Geometry check sheet. Reference: the model listing, model coordinates, mm. Coordinates: 2 decimals unless noted, no trailing zeros. Write each loop counter-clockwise with the first axis right and the second up, starting at its lowest first coordinate (ties: lowest second). Pieces come first, ordered by that corner, then holes.
Autodesk Inventor part; units mm, degrees
ref_plane "YZ Plane" through (0, 0, 0) normal (1, 0, 0) x (0, 1, 0)
ref_plane "XZ Plane" through (0, 0, 0) normal (0, 1, 0) x (-1, 0, 0)
ref_plane "XY Plane" through (0, 0, 0) normal (0, 0, 1) x (1, 0, 0)
sketch "스케치2" plane through (0, 0, 0) normal (0, 0, 1) x (1, 0, 0)
  circle A0 centre (0, 0) radius 1
  circle A1 centre (-8.8212, 8.0626) radius 1
  line L0 (-0.6747, -0.7381) -> (-9.4959, 7.3245)
  line L1 (0.6747, 0.7381) -> (-8.1466, 8.8007)
  line L2 (-1.012, -1.1072) -> (-9.8332, 6.9554)
  line L3 (1.012, 1.1072) -> (-7.8092, 9.1698)
  circle A2 centre (0, 0) radius 1.5
  circle A3 centre (-8.8212, 8.0626) radius 1.5
  dimension "d0" = 0.5
  dimension "d1" = 0.5
  dimension "d2" = 0.5
  dimension "d3" = 0.5
extrude "돌출1" add sketch "스케치2" against normal blind 1 contours A0 L1 A2 L0 | L1 A3 L3 A2 | A2 L2 A3 L0 | L1 A1 L0 A3 picked at (0.2294, 1.2405) picked at (-9.0506, 6.8221)
properties part number "슬롯"
1. Thickness scan on line 1 along X through (y, z) = (0.5, -0.05); line 2 along X through (y, z) = (3, -0.2); line 3 along Y through (x, z) = (-6, -0.5). Record the ranges inside material, lowest first.
Computed values:
line 1: x = -2.77 to -2.03, 0.87 to 1.41
line 2: x = -5.51 to -4.76, -1.8 to -1.06
line 3: y = 3.45 to 4.13, 6.84 to 7.52
2. Sectioned sample at B-B, the plane z = -0.5. Record the boundary of the cut face in (x, y).
Computed values:
outline: (-9.83, 6.96) - (-1.01, -1.11) arc R1.5 ccw to (1.01, 1.11) - (-7.81, 9.17) arc R1.5 ccw to start; hole (-9.5, 7.32) - (-0.67, -0.74) arc R1 ccw to (0.67, 0.74) - (-8.15, 8.8) arc R1 ccw to start
3. Draft check along X on faces 1 (the flat face through (-5.361, 2.868, -0.493)), 2 (the cylindrical face through (-9.906, 9.099, -0.493)), 3 (the cylindrical face through (-9.544, 8.753, -0.493)). Enter one of: released by +X, released by -X, zero draft, split by the parting line, or undercut.
Computed values:
face 1: released by -X
face 2: split by the parting line
face 3: undercut
4. Sectioned sample at C-C, the plane y = 4. Record the boundary of the cut face in (x, z), and give its area (3 significant figures).
Computed values:
outline: (-6.6, -1) - (-5.86, -1) - (-5.86, 0) - (-6.6, 0) - close; (-2.89, -1) - (-2.15, -1) - (-2.15, 0) - (-2.89, 0) - close
area: 1.48 mm2
5. Gauge pin test, flat end, axial feed: pin 1 Ø6 at (x, y) = (-1.5, 6.5) entering from -Z. Record the tip position at first contact, or that the pin passes through.
Computed values:
pin 1: stops at z = -1
6. Sectioned sample at A-A, the plane x = -8.5. Record the boundary of the cut face in (y, z).
Computed values:
outline: (5.74, -1) - (6.41, -1) - (6.41, 0) - (5.74, 0) - close; (9.01, -1) - (9.53, -1) - (9.53, 0) - (9.01, 0) - close
